```python
from build123d import *

# Parameters (mm, degrees)
SKETCH1_W           = 28.956
SKETCH1_H           = 28.956
SKETCH1_R           = 4.445
BOSS_EXTRUDE1_DEPTH = 3.175
SKETCH2_R           = 0.889
CUT_EXTRUDE1_DEPTH  = 4.175
SKETCH3_R           = 6.44921875
BOSS_EXTRUDE2_DEPTH = 6.35
SKETCH4_R           = 3.3528
CUT_EXTRUDE2_DEPTH  = 7.35


with BuildPart() as part:
    # Sketch1 → Boss-Extrude1 (new body)
    with BuildSketch(Plane.XY):
        with Locations((14.478, 14.478)):
            Rectangle(SKETCH1_W, SKETCH1_H)
        with Locations((14.478, 14.478)):
            Circle(SKETCH1_R, mode=Mode.SUBTRACT)
    extrude(amount=BOSS_EXTRUDE1_DEPTH)

    # Sketch2 → Cut-Extrude1 (cut, through all)
    with BuildSketch(Plane.XY.offset(3.175)):
        with Locations((2.11455, 2.11455)):
            Circle(SKETCH2_R)
        with Locations((26.84145, 2.11455)):
            Circle(SKETCH2_R)
        with Locations((26.84145, 26.84145)):
            Circle(SKETCH2_R)
        with Locations((2.11455, 26.84145)):
            Circle(SKETCH2_R)
    extrude(amount=-CUT_EXTRUDE1_DEPTH, mode=Mode.SUBTRACT)

    # Sketch3 → Boss-Extrude2 (add)
    with BuildSketch(Plane.XY.offset(3.175)):
        with Locations((28.956, 14.478)):
            Circle(SKETCH3_R)
    extrude(amount=-BOSS_EXTRUDE2_DEPTH)

    # Sketch4 → Cut-Extrude2 (cut, through all)
    with BuildSketch(Plane.XY.offset(3.175)):
        with Locations((28.956, 14.478)):
            Circle(SKETCH4_R)
    extrude(amount=-CUT_EXTRUDE2_DEPTH, mode=Mode.SUBTRACT)


solid = part.part
```
Verification items for the finished model (mm, model axes). A direction names the side the tool comes from. Give positions to 0.01 mm unless a question says otherwise; leave off trailing zeros. Order: outer loops, then holes, each group sorted by start corner. A loop starts at its lowest first (then second) coordinate and runs counter-clockwise, first axis right, second up. Notation, with made-up numbers: (26, 25) -> (61, 25) arc R28 cw to (61, 53) -> close; hole circle Ø9 at (67.5, 53.5). An arc over 180 degrees is marked (long way). One line per item, written item: value.
(1) Sectioned sample at A-A on x = 13.5. Record the cut outline in (y, z) (3 decimals), then the cut area to 3 significant figures.
Final values:
outline: (0, 0) -> (10.142, 0) -> (10.142, 3.175) -> (0, 3.175) -> close; (18.814, 0) -> (28.956, 0) -> (28.956, 3.175) -> (18.814, 3.175) -> close
area: 64.4 mm^2
(2) Sectioned sample at C-C on z = 2.5. Record the cut outline in (x, y) (3 decimals), then the cut area to 3 significant figures.
Final values:
outline: (0, 0) -> (28.956, 0) -> (28.956, 8.029) arc R6.449 ccw to (28.956, 20.927) -> (28.956, 28.956) -> (0, 28.956) -> close; hole circle Ø1.778 at (2.115, 2.115); hole circle Ø1.778 at (2.115, 26.841); hole circle Ø8.89 at (14.478, 14.478); hole circle Ø6.706 at (28.956, 14.478); hole circle Ø1.778 at (26.841, 2.115); hole circle Ø1.778 at (26.841, 26.841)
area: 796 mm^2
(3) Draft check along Y on faces 1 (the face through (32, 12, -3.175)), 2 (the face through (14, 0, 2)), 3 (the face through (2.962, 2.382, 1.61)). Enter one of: pulls with the +Y half, pulls with the -Y half, needs draft (parallel to the pull), parting line crosses it, or undercut.
Final values:
face 1: needs draft
face 2: pulls with the -Y half
face 3: undercut
(4) Tool access check on faces 4 (the face through (35.107, 16.415, -0.661)), 5 (the face through (28.956, 4, 2)), 6 (the face through (28.956, 25, 2)). Record the directions out of +Z, -Z, +X, -X, +Y, -Y that give a thin tool (end or side, any length) a straight path to the whole face; none if there is none.
Final values:
face 4: -Z
face 5: +Z, -Z, +X, -Y
face 6: +Z, -Z, +X, +Y
(5) Gauge pin test, flat ends, axial feed: pin 1 (1 mm diameter, centred on x = 26, z = -2, fed in from -Y); pin 2 (8.5 mm diameter, centred on x = 15.5, y = 12, fed in from -Z); pin 3 (1 mm diameter, centred on x = 28, z = -1, fed in from +Y); pin 4 (1.6 mm diameter, centred on x = 26.84, y = 2.11, fed in from -Z). Record the tip position at first contact, or that the pin passes through.
Final values:
pin 1: y = 8.51
pin 2: z = 0
pin 3: y = 20.91
pin 4: through
(6) Sectioned sample at B-B on y = 10.5. Record the cut outline in (x, z) (3 decimals), then the cut area to 3 significant figures.
Final values:
outline: (0, 0) -> (12.495, 0) -> (12.495, 3.175) -> (0, 3.175) -> close; (16.461, 0) -> (23.88, 0) -> (23.88, -3.175) -> (34.032, -3.175) -> (34.032, 3.175) -> (16.461, 3.175) -> close
area: 128 mm^2
(7) Scan lines: line 1 along X through (y, z) = (26.75, 2.5); line 2 along X through (y, z) = (12.25, 1.75); line 3 along Z through (x, y) = (15, 20.75) (3 decimals). Record each from-to range of solid material in increasing order. Write a range as [from, to].
Final values:
line 1: [0, 1.23], [3, 25.96], [27.73, 28.96]
line 2: [0, 10.63], [18.32, 26.45], [31.46, 35.01]
line 3: [0, 3.175]
(8) Sectioned sample at D-D on y = 2.5. Record the cut outline in (x, z) (3 decimals), then the cut area to 3 significant figures.
Final values:
outline: (0, 0) -> (1.313, 0) -> (1.313, 3.175) -> (0, 3.175) -> close; (2.916, 0) -> (26.04, 0) -> (26.04, 3.175) -> (2.916, 3.175) -> close; (27.643, 0) -> (28.956, 0) -> (28.956, 3.175) -> (27.643, 3.175) -> close
area: 81.8 mm^2
